Geometry check sheet. Reference: the model listing, model coordinates, mm. A direction names the side the tool comes from. Coordinates: 2 decimals unless noted, no trailing zeros. Write each loop counter-clockwise with the first axis right and the second up, starting at its lowest first coordinate (ties: lowest second). Pieces come first, ordered by that corner, then holes. Notation, with made-up numbers: (-20, 78) -> (27, 78) arc R25 cw to (27, 111) -> close; hole circle Ø1 at (38, 68.5). An arc over 180 degrees is marked (long way). Answer in a Markdown table with one row per item. Add a question column.
1. Cross-section at B-B on y = 3.2. Give the number of separate pieces and of enclosed holes in the cut face, and give its area (3 significant figures).
2. Set-up check for faces 4 (the cylindrical face through (-12.727, 2.535, 0.358)), 5 (the flat face through (165, 2, -10)): record each of +Z, -Z, +X, -X, +Y, -Y from which the full face is reachable in a straight line by a thin tool's end or side.
3. Scan lines: L1, parallel to X at y = 2.4, z = 0; L2, parallel to Z at x = 5, y = 2.95; L3, parallel to Z at x = 175, y = 4. Record each from-to range of solid material in increasing order. Write a range as from..to.
4. Mould release check, pull along X, two halves, no side actions. Record for faces 1 (the cylindrical face through (7.44, 2.54, -9.93)), 2 (the flat face through (165, 2, 10)), 3 (the cylindrical face through (185, 2, 0)): pulls with the +X half, pulls with the -X half, needs draft (parallel to the pull), parting line crosses it, or undercut.
5. Cross-section at A-A on x = -10. Record the cut outline in (y, z), and give its area (3 significant figures).
6. Depth check by flat-ended pin: P1, Ø5, axis at x = 175, z = 0, coming from the +Y side; P2, Ø1, axis at y = 3, z = 6.5, coming from the +X side. Enter the tip coordinate at first touch or a pass-through.
Autodesk Inventor part; units mm, degrees
ref_plane "YZ Plane" through (0, 0, 0) normal (1, 0, 0) x (0, 1, 0)
ref_plane "XZ Plane" through (0, 0, 0) normal (0, 1, 0) x (-1, 0, 0)
ref_plane "XY Plane" through (0, 0, 0) normal (0, 0, 1) x (1, 0, 0)
sketch "Sketch2" plane through (0, 0, 0) normal (0, 1, 0) x (-1, 0, 0)
  circle A0 centre (0, 0) radius 16
  circle A1 centre (-175, 0) radius 10
  line L0 (0, 0) -> (-175, 0)
  line L1 (0, 16) -> (-20, 16)
  line L2 (-175, 10) -> (-155, 10)
  spline S0 degree 4 poles (-20, 16) (-36.9, 16) (-70.7, 16) (-104.3, 10) (-138.1, 10) (-155, 10) knots 0 0 0 0 0 0.5 1 1 1 1 1
  line L3 (0, 0) -> (0, 16) construction
  line L4 (-175, 0) -> (-175, 10) construction
  line L5 (0, -16) -> (-20, -16)
  line L6 (-175, -10) -> (-155, -10)
  spline S1 degree 4 poles (-20, -16) (-36.9, -16) (-70.7, -16) (-104.3, -10) (-138.1, -10) (-155, -10) knots 0 0 0 0 0 0.5 1 1 1 1 1
  line L7 (0, 0) -> (10, 0) construction
  point P0 (0, -16)
  point P1 (-5, 8.6603)
  point P2 (-5, -8.6603)
  dimension "d0" = 32
  dimension "d1" = 20
  dimension "d2" = 175
  dimension "d3" = 20
  dimension "d4" = 20
  dimension "d26" = 10
  dimension "d29" = 360
extrude "Extrusion1" add sketch "Sketch2" along normal blind 5
hole "Hole1" at (-10, 0, 0) at (5, 0, 8.6603) at (5, 0, -8.6603) direction (0, 1, 0) diameter 5.5 end through all
hole "Hole2" at (175, 0, 0) at (0, 0, 0) direction (0, 1, 0) diameter 5.5 end through all
properties part number "RT_ARM_MC_002" material "CFRP"
Results found:
| question | item | result |
|---|---|---|
| 1 | separate pieces | 1 |
| 1 | enclosed holes | 5 |
| 1 | area | 4,990 mm^2 |
| 2 | face 4 | +Y, -Y |
| 2 | face 5 | -Z, +X, +Y, -Y |
| 3 | L1 | x = -16..-12.75, -7.25..-2.75, 2.75..172.25, 177.75..185 |
| 3 | L2 | z = -16..-11.41, -5.91..5.91, 11.41..16 |
| 3 | L3 | z = -10..-2.75, 2.75..10 |
| 4 | face 1 | undercut |
| 4 | face 2 | needs draft |
| 4 | face 3 | pulls with the +X half |
| 5 | outline | (0, -12.49) -> (5, -12.49) -> (5, -2.75) -> (0, -2.75) -> close; (0, 2.75) -> (5, 2.75) -> (5, 12.49) -> (0, 12.49) -> close |
| 5 | area | 97.4 mm^2 |
| 6 | P1 | passes through |
| 6 | P2 | stops at x = 183 |
